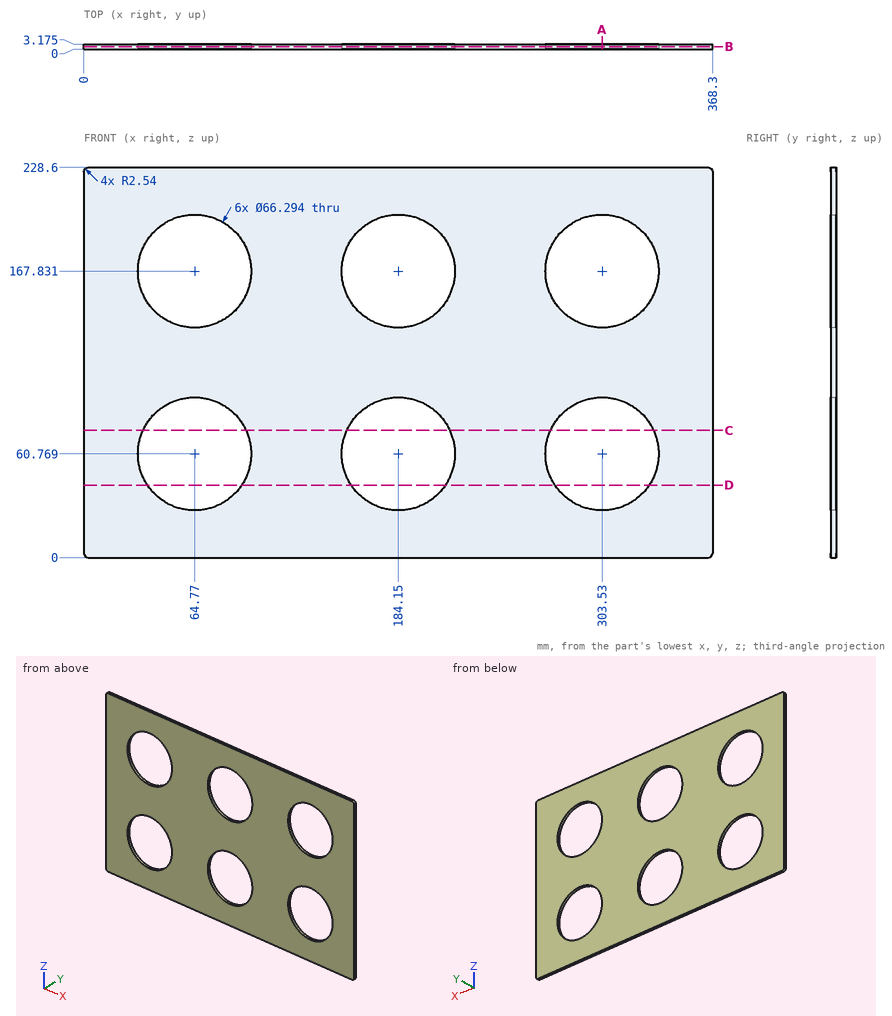
Print and shaded views of the part. All mm, measured from the part's lowest x, y and z. Coordinates: 2 decimals unless noted, no trailing zeros. Order: outer loops, then holes, each group sorted by start corner. A loop starts at its lowest first (then second) coordinate and runs counter-clockwise, first axis right, second up. Notation, with made-up numbers: M 89.25,-19.5 L 118.25,-19.5 A9 ccw 118.25,-12.5 Z; hole C 68,-14.75 d4. An arc over 180 degrees is marked long. One line per question, with ' | ' between items. Start each with the question number.
Q1. Saw through at C-C (z = 74.5). List the corners of the cut face in (x, y) (1 decimal).
Q2. Saw through at A-A (x = 303.53). List the corners of the cut face in (y, z) (1 decimal), then the cut area to 3 significant figures.
Q3. Probe L1, parallel to Z at x = 281, y = 2.6 (1 decimal); L2, parallel to Z at x = 63, y = 0.95; L3, parallel to X at y = 0.65, z = 160. List the from-to ranges inside material, lowest first. Write a range as from..to.
Q4. Saw through at D-D (z = 42.5). List the corners of the cut face in (x, y) (1 decimal).
Q5. Saw through at B-B (y = 1.6). Count the separate pieces of the cut face and the enclosed holes in it, then the cut area to 3 significant figures.
Check values:
1) outline: M 0,0 L 34.6,0 L 34.6,3.2 L 0,3.2 Z; M 94.9,0 L 154,0 L 154,3.2 L 94.9,3.2 Z; M 214.3,0 L 273.4,0 L 273.4,3.2 L 214.3,3.2 Z; M 333.7,0 L 368.3,0 L 368.3,3.2 L 333.7,3.2 Z
2) outline: M 0,0 L 3.2,0 L 3.2,27.6 L 0,27.6 Z; M 0,93.9 L 3.2,93.9 L 3.2,134.7 L 0,134.7 Z; M 0,201 L 3.2,201 L 3.2,228.6 L 0,228.6 Z | area: 305 mm2
3) L1: z = 0..36.5, 85.1..143.5, 192.1..228.6 | L2: z = 0..27.67, 93.87..134.73, 200.93..228.6 | L3: x = 0..32.56, 96.98..151.94, 216.36..271.32, 335.74..368.3
4) outline: M 0,0 L 37.1,0 L 37.1,3.2 L 0,3.2 Z; M 92.4,0 L 156.5,0 L 156.5,3.2 L 92.4,3.2 Z; M 211.8,0 L 275.9,0 L 275.9,3.2 L 211.8,3.2 Z; M 331.2,0 L 368.3,0 L 368.3,3.2 L 331.2,3.2 Z
5) separate pieces: 1 | enclosed holes: 6 | area: 63,500 mm2
